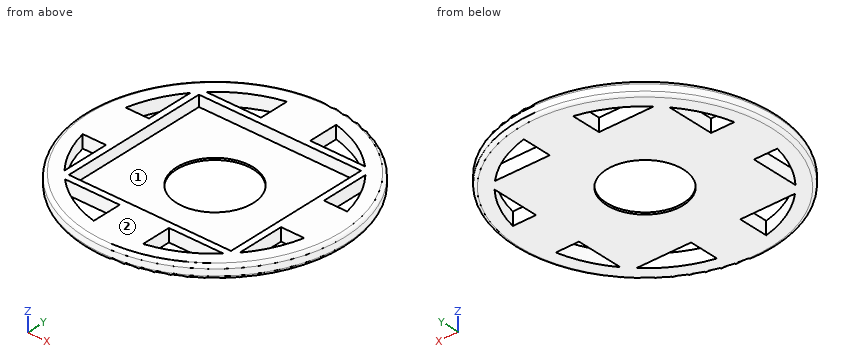
from build123d import *

# Parameters (mm, degrees)
F0_R     = 10
F1_DEPTH = 1
F2_W     = 12.5
F2_H     = 11.5
F3_DEPTH = 0.85
F5_R     = 2.9508175635
F6_DEPTH = 0.15
F7_R     = 0.25
F9_DEPTH = 1


# Not quite as in the source:
# - a feature names something its author has since deleted; it is built from what else it names


with BuildPart() as f1:
    # F0 (on Top) → F1 (new body)
    with BuildSketch(Plane.XY):
        Circle(F0_R)
    extrude(amount=F1_DEPTH)

    # F2 (on face) → F3 (cut)
    with BuildSketch(Plane.XY.offset(1)):
        with Locations((0, 0.0005259759)):
            Rectangle(F2_W, F2_H)
    extrude(amount=-F3_DEPTH, mode=Mode.SUBTRACT)

    # F5 (on offset) → F6 (cut)
    with BuildSketch(Plane.XY.offset(0.15)):
        Circle(F5_R)
    extrude(amount=-F6_DEPTH, mode=Mode.SUBTRACT)

    # F7
    f7_edges = [f1.edges().sort_by_distance(p)[0] for p in [
        (-10, 0, 1),
        (-10, 0, 0),
    ]]
    fillet(f7_edges, radius=F7_R)

    # F8 (on face) → F9 (cut, through all)
    with BuildSketch(Plane.XY.offset(1)):
        with BuildLine():
            Line((1.9, 8.5412235657), (1.9, 6.2505259759))
            Line((1.9, 6.2505259759), (6.1231874889, 6.2505259759))
            ThreePointArc((6.1231874889, 6.2505259759), (4.1718950409, 7.6914102587), (1.9, 8.5412235657))
        make_face()
        with BuildLine():
            Line((-6.75, 1.9), (-6.75, 5.5677643628))
            ThreePointArc((-6.75, 5.5677643628), (-7.8624743809, 3.8397912196), (-8.5412235657, 1.9))
            Line((-8.5412235657, 1.9), (-6.75, 1.9))
        make_face()
        with BuildLine():
            Line((-6.75, -5.5677643628), (-6.75, -1.9))
            Line((-6.75, -1.9), (-8.5412235657, -1.9))
            ThreePointArc((-8.5412235657, -1.9), (-7.8624743809, -3.8397912196), (-6.75, -5.5677643628))
        make_face()
        with BuildLine():
            Line((-1.9, -6.2505259759), (-6.1231874889, -6.2505259759))
            ThreePointArc((-6.1231874889, -6.2505259759), (-4.1718950409, -7.6914102587), (-1.9, -8.5412235657))
            Line((-1.9, -8.5412235657), (-1.9, -6.2505259759))
        make_face()
        with BuildLine():
            ThreePointArc((1.9, -8.5412235657), (4.1718950409, -7.6914102587), (6.1231874889, -6.2505259759))
            Line((6.1231874889, -6.2505259759), (1.9, -6.2505259759))
            Line((1.9, -6.2505259759), (1.9, -8.5412235657))
        make_face()
        with BuildLine():
            Line((8.5412235657, -1.9), (6.75, -1.9))
            Line((6.75, -1.9), (6.75, -5.5677643628))
            ThreePointArc((6.75, -5.5677643628), (7.8624743809, -3.8397912196), (8.5412235657, -1.9))
        make_face()
        with BuildLine():
            ThreePointArc((8.5412235657, 1.9), (7.8624743809, 3.8397912196), (6.75, 5.5677643628))
            Line((6.75, 5.5677643628), (6.75, 1.9))
            Line((6.75, 1.9), (8.5412235657, 1.9))
        make_face()
        with BuildLine():
            Line((-6.1231874889, 6.2505259759), (-1.9, 6.2505259759))
            Line((-1.9, 6.2505259759), (-1.9, 8.5412235657))
            ThreePointArc((-1.9, 8.5412235657), (-4.1718950409, 7.6914102587), (-6.1231874889, 6.2505259759))
        make_face()
    extrude(amount=-F9_DEPTH, mode=Mode.SUBTRACT)


solid = f1.part
Here's how the part is built. I have some questions about the finished solid (model axes, mm). Face numbers are marked on the shaded views. Give positions to 0.01 mm unless a question says otherwise; leave off trailing zeros. Order: outer loops, then holes, each group sorted by start corner. A loop starts at its lowest first (then second) coordinate and runs counter-clockwise, first axis right, second up. Notation, with made-up numbers: (-37, 69) -> (8, 69) arc R26 cw to (8, 102) -> close; hole circle Ø10 at (54.5, -8.5). An arc over 180 degrees is marked (long way). Use a Markdown table: item, result. Add a question column.
Item 1: Imagine slicing it at C-C on z = 0.5. Give the number of separate pieces and of enclosed holes in the cut face, plus the area to 3 significant figures.
Item 2: Will these pins go through, and if not, where does the flat tip stop? pin 1 (0.5 mm diameter, centred on y = -3.5, z = 0.5, fed in from -X); pin 2 (5 mm diameter, centred on x = -0.5, y = -1.5, fed in from +Z); pin 3 (0.5 mm diameter, centred on x = 3, z = 0.5, fed in from -Y).
Item 3: If we mould it in two halves opening along X, with no side actions, what happens to the marked faces 1 and 2? For each: pulls with the +X half, pulls with the -X half, needs draft (parallel to the pull), parting line crosses it, or undercut.
Item 4: I need wall thicknesses on line 1 (X direction, y = 5.25, z = 0.7); line 2 (Y direction, x = 5, z = 0.1); line 3 (Y direction, x = -2.75, z = 0.75). Which ranges of each line are inside material? Lowest first, please.
Item 5: Imagine slicing it at A-A on x = 0. Please give me the cut outline in (y, z), plus the area to 3 significant figures.
Item 6: Imagine slicing it at B-B on y = 0. Please give me the cut outline in (x, z).
Data:
| question | item | result |
|---|---|---|
| 1 | separate pieces | 1 |
| 1 | enclosed holes | 9 |
| 1 | area | 131 mm² |
| 2 | pin 1 | stops at x = -9.46 |
| 2 | pin 2 | stops at z = 0.15 |
| 2 | pin 3 | stops at y = -9.61 |
| 3 | face 1 | undercut |
| 3 | face 2 | needs draft |
| 4 | line 1 | x = -8.51 to -7, -6.75 to -6.25, 6.25 to 6.75, 7 to 8.51 |
| 4 | line 2 | y = -8.6 to -7.18, -6.25 to 6.25, 7.18 to 8.6 |
| 4 | line 3 | y = -9.61 to -8.31, -6.25 to -5.75, 5.75 to 6.25, 8.31 to 9.61 |
| 5 | outline | (-10, 0.25) arc R0.25 ccw to (-9.75, 0) -> (-2.95, 0) -> (-2.95, 0.15) -> (-5.75, 0.15) -> (-5.75, 1) -> (-9.75, 1) arc R0.25 ccw to (-10, 0.75) -> close; (2.95, 0) -> (9.75, 0) arc R0.25 ccw to (10, 0.25) -> (10, 0.75) arc R0.25 ccw to (9.75, 1) -> (5.75, 1) -> (5.75, 0.15) -> (2.95, 0.15) -> close |
| 5 | area | 9.29 mm² |
| 6 | outline | (-10, 0.25) arc R0.25 ccw to (-9.75, 0) -> (-2.95, 0) -> (-2.95, 0.15) -> (-6.25, 0.15) -> (-6.25, 1) -> (-9.75, 1) arc R0.25 ccw to (-10, 0.75) -> close; (2.95, 0) -> (9.75, 0) arc R0.25 ccw to (10, 0.25) -> (10, 0.75) arc R0.25 ccw to (9.75, 1) -> (6.25, 1) -> (6.25, 0.15) -> (2.95, 0.15) -> close |
